from build123d import *

# Parameters (mm, degrees)
SKETCH1_R           = 16.15
SKETCH1_R_2         = 11.15
BOSS_EXTRUDE1_DEPTH = 60
BOSS_EXTRUDE2_START = 5
SKETCH2_R           = 16.15
BOSS_EXTRUDE2_DEPTH = 5
FILLET1_R           = 1


with BuildPart() as part:
    # Sketch1 → Boss-Extrude1 (new body)
    with BuildSketch(Plane(origin=(0, 0, 0), x_dir=(1, 0, 0), z_dir=(0, 1, 0))):
        with Locations(Location((0, 0, 0), (0, 0, 270))):
            Circle(SKETCH1_R)
        with Locations(Location((0, 0, 0), (0, 0, 270))):
            Circle(SKETCH1_R_2, mode=Mode.SUBTRACT)
    extrude(amount=BOSS_EXTRUDE1_DEPTH)

    # Sketch2 → Boss-Extrude2 (add)
    with BuildSketch(Plane.XZ.offset(BOSS_EXTRUDE2_START)):
        with Locations(Location((0, 0, 0), (0, 0, 270))):
            Circle(SKETCH2_R)
    extrude(amount=-BOSS_EXTRUDE2_DEPTH)

    # Sketch3 → Revolve1 (revolve)
    with BuildSketch(Plane.XY, mode=Mode.PRIVATE) as revolve1_sk:
        Polygon((-11.15, 60), (-5, 65), (-5, 70), (-16.15, 70), (-16.15, 60), align=None)
    revolve(revolve1_sk.sketch.rotate(Axis((0, 60, 0), (0, -1, 0)), 270), axis=Axis((0, 60, 0), (0, -1, 0)))

    # Fillet1
    fillet1_edges = [part.edges().sort_by_distance(p)[0] for p in [
        (0, 70, -16.15),
        (0, -5, 16.15),
    ]]
    fillet(fillet1_edges, radius=FILLET1_R)


solid = part.part
Geometry: final body of the model. Coordinates: model frame, mm. A direction names the side the tool comes from. Coordinates: 2 decimals unless noted, no trailing zeros. Loops run counter-clockwise (first coordinate to the right, second up) from the corner with the lowest first, then second, coordinate; pieces in that order, holes last. Notation, with made-up numbers: M 8,64 L 61,64 A26 ccw 61,79 Z; hole C 71,21 d11. An arc over 180 degrees is marked long. One line per item, written item: value. Start each with the question number.
1) Draft query along X for faces 1 (the conical face through (-5.25, 64.76, -0.69)), 2 (the cylindrical face through (-10.885, 29.58, -2.417)), 3 (the flat face through (0, -5, 0)). Return one class per face: released by +X, released by -X, zero draft, split by the parting line, or undercut.
2) Reachability of faces 4 (the flat face through (0, 0, 0)), 5 (the cylindrical face through (4.88, 67.54, -1.08)), 6 (the flat face through (-4, 70, 4)) from +Z, -Z, +X, -X, +Y, -Y: full face, straight path, thin tool, end or side. Return the list, or none.
3) Cut plane A-A (x = 0). Return loops of the section in (y, z).
4) Pin query (flat end, axial travel): P1, Ø6, axis at x = 0, z = 0, coming from the +Y side; P2, Ø3, axis at y = 61.5, z = -10.5, coming from the +X side; P3, Ø5, axis at x = -8, y = 20.5, coming from the -Z side. Return the tip coordinate at first contact, or that it passes through.
5) Cut plane B-B (z = 0). Return loops of the section in (x, y).
6) Cut plane C-C (y = 32). Return loops of the section in (x, z).
7) Material intervals for L1, parallel to X at y = 29, z = 0; L2, parallel to X at y = 68.15, z = 0; L3, parallel to Z at x = 4, y = 67, sorted ascending. Write a range as from..to.
Evaluation:
1. face 1: undercut
1. face 2: undercut
1. face 3: zero draft
2. face 4: none
2. face 5: +Y
2. face 6: +Z, -Z, +X, -X, +Y
3. outline: M -5,-15.15 A1 ccw -4,-16.15 L 69,-16.15 A1 ccw 70,-15.15 L 70,-5 L 65,-5 L 60,-11.15 L 0,-11.15 L 0,11.15 L 60,11.15 L 65,5 L 70,5 L 70,15.15 A1 ccw 69,16.15 L -4,16.15 A1 ccw -5,15.15 Z
4. P1: y = 0
4. P2: x = 13.41
4. P3: z = -15.18
5. outline: M -16.15,-4 A1 ccw -15.15,-5 L 15.15,-5 A1 ccw 16.15,-4 L 16.15,69 A1 ccw 15.15,70 L 5,70 L 5,65 L 11.15,60 L 11.15,0 L -11.15,0 L -11.15,60 L -5,65 L -5,70 L -15.15,70 A1 ccw -16.15,69 Z
6. outline: C 0,0 d32.3; hole C 0,0 d22.3
7. L1: -16.15..-11.15, 11.15..16.15
7. L2: -16.15..-5, 5..16.15
7. L3: -15.65..-3, 3..15.65
